Work out the finished part from the listing and answer in its coordinate system (mm). A direction names the side the tool comes from. Coordinates: 2 decimals unless noted, no trailing zeros. Loops run counter-clockwise (first coordinate to the right, second up) from the corner with the lowest first, then second, coordinate; pieces in that order, holes last. Notation, with made-up numbers: (-16, 42.5) -> (-11, 42.5) arc R31 ccw to (-11, 76.5) -> close; hole circle Ø8 at (78, 53.5). An arc over 180 degrees is marked (long way). One line per question, with ' | ' between items.
```python
from build123d import *

# Parameters (mm, degrees)
F1_DEPTH       = 12
F5_DEPTH       = 19.9
F7_R           = 11.5
F8_DEPTH       = 8
F11_ANGLE_BACK = 20
F11_ANGLE      = 40


with BuildPart() as f1:
    # F0 (on Top) → F1 (new body)
    with BuildSketch(Plane.XY):
        with BuildLine():
            Line((0, 0), (-20, 0))
            ThreePointArc((-20, 0), (-22, 2), (-20, 4))
            Line((-20, 4), (-8, 4))
            Line((-8, 4), (-8, 7))
            Line((-8, 7), (-20, 7))
            ThreePointArc((-20, 7), (-25, 2), (-20, -3))
            Line((-20, -3), (0, -3))
            ThreePointArc((0, -3), (5, 2), (0, 7))
            Line((0, 7), (-3, 7))
            Line((-3, 7), (-3, 4))
            Line((-3, 4), (0, 4))
            ThreePointArc((0, 4), (2, 2), (0, 0))
        make_face()
    extrude(amount=F1_DEPTH)

    # F4 (on line) → F5 (join)
    with BuildSketch(Plane(origin=(-14.7844431916, 0, -7.9443702008), x_dir=(0, -1, 0), z_dir=(-0.8808807435, 0, -0.4733382677))):
        Polygon((3, 11.0186671228), (3, 9.0186671228), (5.3, 9.0186671228), (5.3, 11.0186671228), (6.1, 11.0186671228), (6.1, 9.0186671228), (6.9, 9.0186671228), (6.9, 11.8186671228), (4.5, 11.8186671228), (4.5, 11.0186671228), align=None)
    extrude(amount=-F5_DEPTH)

    # F7 (on offset) → F8 (join)
    with BuildSketch(Plane(origin=(-1.5712320387, 0, -0.8442961852), x_dir=(0, -1, 0), z_dir=(-0.8808807435, 0, -0.4733382677))):
        with BuildLine():
            ThreePointArc((34, 9.6230288318), (22.5099800796, 23.3961911411), (6.9, 14.5616521217))
            Line((6.9, 14.5616521217), (6.9, 4.6844055418))
            ThreePointArc((6.9, 4.6844055418), (22.5099800796, -4.1501334776), (34, 9.6230288318))
        make_face()
        with Locations((20, 9.6230288318)):
            Circle(F7_R, mode=Mode.SUBTRACT)
        with BuildLine():
            Line((6.9, 4.6844055418), (6.9, 14.5616521217))
            ThreePointArc((6.9, 14.5616521217), (6, 9.6230288318), (6.9, 4.6844055418))
        make_face()
    extrude(amount=F8_DEPTH)

    # F10 (on offset) → F11 (revolve)
    with BuildSketch(Plane.XZ.offset(20), mode=Mode.PRIVATE) as f11_sk:
        Polygon((-6.7922217721, -8.029286104), (-7.7298357056, -6.2843900851), (-11.4623919126, -7.7224527269), align=None)
        Polygon((-21.8758338022, 11.6569236308), (-18.6166158629, 13.9758670161), (-19.5542297964, 15.720763035), align=None)
    revolve(f11_sk.sketch.rotate(Axis((-15.3602525801, -20, 2.6705470646), (-0.8808807435, 0, -0.4733382677)), -F11_ANGLE_BACK), axis=Axis((-15.3602525801, -20, 2.6705470646), (-0.8808807435, 0, -0.4733382677)), revolution_arc=F11_ANGLE)


solid = f1.part
```
1) Find section A-A (y = 2). Write down the section's boundary in (x, z), plus the area to 3 significant figures.
Check values:
outline: (-25, 0) -> (-22, 0) -> (-22, 12) -> (-25, 12) -> close; (2, 0) -> (5, 0) -> (5, 12) -> (2, 12) -> close | area: 72.0 mm^2
2) Flat-ended cylindrical pins translate along their axes: pin 1 (3.5 mm diameter, centred on y = 5.5, z = 8, fed in from +X); pin 2 (1.7 mm diameter, centred on x = -17.5, z = 3.5, fed in from -Y); pin 3 (10 mm diameter, centred on y = -22.5, z = 8.5, fed in from +X); pin 4 (8 mm diameter, centred on x = -4.5, z = 14.5, fed in from +Y). Find the tip coordinate at first contact, or state that the pin passes through.
Check values:
pin 1: stops at x = 4.68 | pin 2: stops at y = -6.9 | pin 3: stops at x = -18.39 | pin 4: stops at y = 7
3) For faces 1 (the face through (-4, -6.9, 9)), 2 (the face through (-10.2, -0.2, 0)), 3 (the face through (-2, 4, 6)), 4 (the face through (-10.2, -0.2, 12)), determine the directions among +Z, -Z, +X, -X, +Y, -Y from which every point of the face is accessible in a straight line to the end or side of a thin tool.
Check values:
face 1: +Z, +X, -Y | face 2: -Z, +X, -X, +Y | face 3: +Z, -Z | face 4: +Z, +X, -X, +Y
4) The mould has two halves that part along X. Classify faces 5 (the face through (-25, 2, 6)), 6 (the face through (-19.788, -24.14, 13.206)), 7 (the face through (-19.6, -3, 0.7)): released by +X, released by -X, zero draft, split by the parting line, or undercut.
Check values:
face 5: released by -X | face 6: undercut | face 7: zero draft
5) Find section D-D (y = -8). Write down the section's boundary in (x, z), plus the area to 3 significant figures.
Check values:
outline: (-16.59, 10.2) -> (-9.76, -2.51) -> (-2.71, 1.28) -> (-9.54, 13.98) -> close | area: 115 mm^2
6) Find the intervals of material crossed by line 1 along Y through (x, z) = (-1.25, 8.5); line 2 along Y through (x, z) = (-6.5, 6); line 3 along Z through (x, y) = (3.25, 1.5), in increasing order.
Check values:
line 1: y = -3 to 0, 4 to 7 | line 2: y = -33.94 to -31.43, -8.57 to -6.06, -3 to 0 | line 3: z = 0 to 12
7) Find section C-C (x = -16.5). State how many separate pieces and enclosed holes the cut face has, plus the area to 3 significant figures.
Check values:
separate pieces: 3 | enclosed holes: 0 | area: 153 mm^2
8) Find section B-B (y = -27.5). Write down the section's boundary in (x, z), plus the area to 3 significant figures.
Check values:
outline: (-18.77, 14.26) -> (-17.3, 11.53) -> (-10.25, 15.31) -> (-11.72, 18.05) -> close; (-9.05, -3.83) -> (-7.58, -6.57) -> (-0.53, -2.78) -> (-2, -0.05) -> close | area: 49.7 mm^2
